Geometry check sheet. Reference: the model listing, model coordinates, mm. Face numbers are marked on the shaded views. Give positions to 0.01 mm unless a question says otherwise; leave off trailing zeros. Write each loop counter-clockwise with the first axis right and the second up, starting at its lowest first coordinate (ties: lowest second). Pieces come first, ordered by that corner, then holes. Notation, with made-up numbers: M 29.25,46.5 L 61.25,46.5 A21 ccw 61.25,82.5 Z; hole C 14,-3.75 d2. An arc over 180 degrees is marked long. Write each question's results on one line, items separated by ' | '.
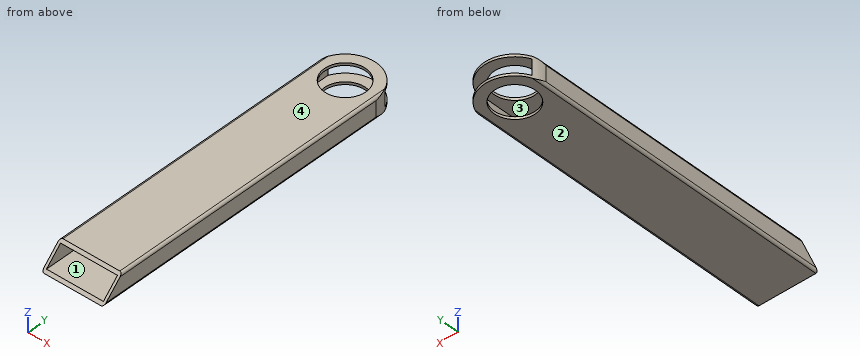
```python
from build123d import *

# Parameters (mm, degrees)
SKETCH1_W           = 34.925
SKETCH1_H           = 9.525
BOSS_EXTRUDE1_DEPTH = 203.2
SKETCH2_R           = 12.7
CUT_EXTRUDE1_DEPTH  = 13.7
CUT_EXTRUDE2_DEPTH  = 39.1000001


with BuildPart() as part:
    # Sketch1 → Boss-Extrude1 (new body)
    with BuildSketch(Plane(origin=(0, 0, 0), x_dir=(1, 0, 0), z_dir=(0, 1, 0))):
        with BuildLine():
            Line((1.5875, 0), (36.5125, 0))
            ThreePointArc((36.5125, 0), (37.635032015, 0.464967985), (38.1, 1.5875))
            Line((38.1, 1.5875), (38.1, 11.1125))
            ThreePointArc((38.1, 11.1125), (37.635032015, 12.235032015), (36.5125, 12.7))
            Line((36.5125, 12.7), (1.5875, 12.7))
            ThreePointArc((1.5875, 12.7), (0.464967985, 12.235032015), (0, 11.1125))
            Line((0, 11.1125), (0, 1.5875))
            ThreePointArc((0, 1.5875), (0.464967985, 0.464967985), (1.5875, 0))
        make_face()
        with Locations((19.05, 6.35)):
            Rectangle(SKETCH1_W, SKETCH1_H, mode=Mode.SUBTRACT)
    extrude(amount=BOSS_EXTRUDE1_DEPTH)

    # Sketch2 → Cut-Extrude1 (cut, through all)
    with BuildSketch(Plane.XY):
        with Locations((19.05, 184.15)):
            Circle(SKETCH2_R)
        with BuildLine():
            Line((0, 184.15), (0, 209.55))
            Line((0, 209.55), (38.1, 209.55))
            Line((38.1, 209.55), (38.1, 184.15))
            ThreePointArc((38.1, 184.15), (19.05, 203.2), (0, 184.15))
        make_face()
    extrude(amount=-CUT_EXTRUDE1_DEPTH, mode=Mode.SUBTRACT)

    # Sketch3 → Cut-Extrude2 (cut, through all)
    with BuildSketch(Plane(origin=(38.1, 0, 0), x_dir=(0, 0, -1), z_dir=(1, 0, 0))):
        Polygon((0, 0), (12.7, 0), (0, 12.7), align=None)
    extrude(amount=-CUT_EXTRUDE2_DEPTH, mode=Mode.SUBTRACT)


solid = part.part
```
Q1. Material ranges on probe 1 along Z at (x, y) = (15, 20); probe 2 along X at (y, z) = (12, -10); probe 3 along X at (y, z) = (183, -0.75), recorded low to high. Write a range as [from, to].
Answer key:
probe 1: z = [-12.7, -11.11], [-1.59, 0] | probe 2: x = [0, 1.59], [36.51, 38.1] | probe 3: x = [0.24, 6.4], [31.7, 37.86]
Q2. Section check D-D (x = 34). Enter the section's corners in (y, z), then the cut area to 3 significant figures.
Answer key:
outline: M 0,-12.7 L 195.96,-12.7 L 195.96,-11.11 L 1.59,-11.11 Z; M 11.11,-1.59 L 195.96,-1.59 L 195.96,0 L 12.7,0 Z | area: 602 mm2
Q3. Section check A-A (z = -6.75). Enter the section's corners in (x, y).
Answer key:
outline: M 0,5.95 L 1.59,5.95 L 1.59,191.76 A19.05 ccw 0,184.15 Z; M 36.51,5.95 L 38.1,5.95 L 38.1,184.15 A19.05 ccw 36.51,191.76 Z
Q4. Section check C-C (x = 19.05). Enter the section's corners in (y, z), then the cut area to 3 significant figures.
Answer key:
outline: M 0,-12.7 L 171.45,-12.7 L 171.45,-11.11 L 1.59,-11.11 Z; M 11.11,-1.59 L 171.45,-1.59 L 171.45,0 L 12.7,0 Z; M 196.85,-12.7 L 203.2,-12.7 L 203.2,-11.11 L 196.85,-11.11 Z; M 196.85,-1.59 L 203.2,-1.59 L 203.2,0 L 196.85,0 Z | area: 544 mm2
Q5. Section check B-B (y = 126). Enter the section's corners in (x, z) (1 decimal).
Answer key:
outline: M 0,-11.1 A1.6 ccw 1.6,-12.7 L 36.5,-12.7 A1.6 ccw 38.1,-11.1 L 38.1,-1.6 A1.6 ccw 36.5,0 L 1.6,0 A1.6 ccw 0,-1.6 Z; hole M 1.6,-11.1 L 36.5,-11.1 L 36.5,-1.6 L 1.6,-1.6 Z
Q6. Release check for a two-part mould opening along Z. For the marked faces 1, 2, 3 and 4 record: released by +Z, released by -Z, zero draft, split by the parting line, or undercut.
Answer key:
face 1: undercut | face 2: released by -Z | face 3: undercut | face 4: released by +Z
